```python
from build123d import *

# Parameters (mm, degrees)
F0_W     = 3
F0_H     = 20
F1_DEPTH = 0.25
F2_W     = 3
F2_H     = 40
F3_DEPTH = 2
F4_W     = 3
F4_H     = 20
F5_DEPTH = 2
F6_DEPTH = 1.5


with BuildPart() as f1:
    # F0 (on Front) → F1 (new body, symmetric)
    with BuildSketch(Plane.XZ):
        with Locations((0, -30)):
            Rectangle(F0_W, F0_H)
    extrude(amount=F1_DEPTH, both=True)

    # F2 (on Front) → F3 (join, symmetric)
    with BuildSketch(Plane.XZ):
        Rectangle(F2_W, F2_H)
    extrude(amount=F3_DEPTH, both=True)

    # F4 (on Front) → F5 (join)
    with BuildSketch(Plane.XZ):
        with Locations((0, 30)):
            Rectangle(F4_W, F4_H)
    extrude(amount=F5_DEPTH)

    # F4 (on Front) → F6 (cut)
    with BuildSketch(Plane.XZ):
        with Locations((0, 30)):
            Rectangle(F4_W, F4_H)
    extrude(amount=F6_DEPTH, mode=Mode.SUBTRACT)


solid = f1.part
```
Verification items for the finished model (mm, model axes). A direction names the side the tool comes from. Round coordinates to 2 decimals unless told otherwise and drop trailing zeros. Write each loop counter-clockwise with the first axis right and the second up, starting at its lowest first coordinate (ties: lowest second). Pieces come first, ordered by that corner, then holes. Notation, with made-up numbers: (6, 69.25) - (28, 69.25) arc R22 cw to (28, 88.25) - close; hole circle Ø7 at (39, 27.25). An arc over 180 degrees is marked (long way). Answer as a JSON object with one key per item and string values. Group by question number.
Q1. Section check A-A, the plane x = -0.15. Enter the section's corners in (y, z).
Q2. Section check C-C, the plane y = 1.25. Enter the section's corners in (x, z), plus the area to 3 significant figures.
Q3. Tool access check on faces 1 (the flat face through (0, -2, 10)), 2 (the flat face through (0, 2, 0)), 3 (the flat face through (0, 0, 20)), 4 (the flat face through (0, 0.25, -30)), 5 (the flat face through (0, -0.25, -30)). Record the directions out of +Z, -Z, +X, -X, +Y, -Y that give a thin tool (end or side, any length) a straight path to the whole face; none if there is none.
Q4. Go/stop test with flat-tipped pins: pin 1 Ø0.9 at (x, z) = (0, -31.5) entering from -Y; pin 2 Ø0.9 at (x, z) = (-0.5, -25.5) entering from +Y; pin 3 Ø1.4 at (x, y) = (0.5, -1.5) entering from -Z. Record where each tip stops, or that it passes through.
Q5. Thickness scan on line 1 (Y direction, x = -1.2, z = -28); line 2 (Z direction, x = 0.8, y = 0.7); line 3 (Y direction, x = 0.05, z = 23). Record the ranges inside material, lowest first.
Q6. Section check B-B, the plane z = -24. Enter the section's corners in (x, y), plus the area to 3 significant figures.
Found:
{
 "1": {"outline": "(-2, -20) - (-0.25, -20) - (-0.25, -40) - (0.25, -40) - (0.25, -20) - (2, -20) - (2, 20) - (-1.5, 20) - (-1.5, 40) - (-2, 40) - close"},
 "2": {"outline": "(-1.5, -20) - (1.5, -20) - (1.5, 20) - (-1.5, 20) - close", "area": "120 mm^2"},
 "3": {"face 1": "+Z, -Z, +X, -X, -Y", "face 2": "+Z, -Z, +X, -X, +Y", "face 3": "+Z, +X, -X, +Y", "face 4": "-Z, +X, -X, +Y", "face 5": "-Z, +X, -X, -Y"},
 "4": {"pin 1": "stops at y = -0.25", "pin 2": "stops at y = 0.25", "pin 3": "stops at z = -20"},
 "5": {"line 1": "y = -0.25 to 0.25", "line 2": "z = -20 to 20", "line 3": "y = -2 to -1.5"},
 "6": {"outline": "(-1.5, -0.25) - (1.5, -0.25) - (1.5, 0.25) - (-1.5, 0.25) - close", "area": "1.50 mm^2"}
}
